Autodesk Inventor part; units mm, degrees
ref_plane "YZ Plane" through (0, 0, 0) normal (1, 0, 0) x (0, 1, 0)
ref_plane "XZ Plane" through (0, 0, 0) normal (0, 1, 0) x (-1, 0, 0)
ref_plane "XY Plane" through (0, 0, 0) normal (0, 0, 1) x (1, 0, 0)
sketch "Sketch1" plane through (0, 0, 0) normal (1, 0, 0) x (0, 1, 0)
  line L0 (0, 3.25) -> (10, 3.25)
  line L1 (10, 3.25) -> (10, -3.25)
  line L2 (10, -3.25) -> (0, -3.25)
  line L3 (0, -3.25) -> (0, 3.25)
  line L4 (10, 1.6898) -> (6.2365, 3.25)
  line L5 (10, -1.7859) -> (6.2365, -3.25)
  point P0 (0, 0)
  dimension "d0" = 10
  dimension "d1" = 6.5
  dimension "d2" = 3.25
  dimension "d3" = 0
extrude "Extrusion1" add sketch "Sketch1" along normal blind 3.9 and the other way blind 1.5 contours L0 L4 L1 L5 L2 L3
sketch "Sketch2" plane through (-1.5, 0, -3.25) normal (0, -1, 0) x (1, 0, 0)
  circle A0 centre (1.5, 3.25) radius 0.425
  line L0 (0, 0) -> (0, 6.5)
  dimension "d7" = 0.85
  dimension "d12" = 1.5
extrude "Extrusion2" add sketch "Sketch2" along normal blind 3.6
sketch "Sketch3" plane through (-1.5, 10, 1.6898) normal (0, 1, 0) x (1, 0, 0)
  circle A0 centre (1.5, 1.6898) radius 0.8517
extrude "Extrusion3" cut sketch "Sketch3" against normal blind 1
sketch "Sketch4" plane through (-1.5, 0, 3.25) normal (0, 0, 1) x (1, 0, 0)
  line L0 (0.648, 5.5866) -> (2.3749, 5.5866)
  line L1 (2.3749, 5.5866) -> (2.3749, 1.0456)
  line L2 (2.3749, 1.0456) -> (0.648, 1.0456)
  line L3 (0.648, 1.0456) -> (0.648, 5.5866)
  point P0 (1.5, 0)
extrude "Extrusion4" cut sketch "Sketch4" against normal blind 1
pattern_linear "Rectangular Pattern1" count 2 spacing 2.54 along (1, 0, 0) of "Extrusion4", "Extrusion3", "Extrusion2"
properties part number "Screw_Terminal_2Pos"
Verification items for the finished model (mm, model axes). A direction names the side the tool comes from. Coordinates: 2 decimals unless noted, no trailing zeros. Order: outer loops, then holes, each group sorted by start corner. A loop starts at its lowest first (then second) coordinate and runs counter-clockwise, first axis right, second up. Notation, with made-up numbers: (-3.5, -38.5) -> (33.5, -38.5) arc R22 ccw to (33.5, -22.5) -> close; hole circle Ø2 at (74, 46). An arc over 180 degrees is marked (long way). Use CSV: the item, a comma, the result in double quotes. Start each with the question number.
Q1. Section check C-C, the plane z = 2.75. Record the cut outline in (x, y).
Q2. Tool access check on faces 1 (the flat face through (2.5, -3.6, 0)), 2 (the flat face through (3.415, 3, 3)). Record the directions out of +Z, -Z, +X, -X, +Y, -Y that give a thin tool (end or side, any length) a straight path to the whole face; none if there is none.
Q3. Depth check by flat-ended pin: P1, Ø0.5, axis at x = 0.5, y = 2, coming from the +Z side; P2, Ø0.8, axis at x = 2.5, z = 2.5, coming from the +Y side; P3, Ø0.8, axis at x = 0, z = 2.5, coming from the -Y side. Enter the tip coordinate at first touch or a pass-through.
Q4. Draft check along Z on faces 3 (the cylindrical face through (2.115, -1.775, -0.019)), 4 (the cylindrical face through (-0.111, 9.507, -0.844)), 5 (the flat face through (3.9, 5, 0)). Enter one of: +Z half, -Z half, draft (parallel to the pull), parting line (faces both ways), or undercut.
Q5. Section check A-A, the plane y = -1.75. Record the cut outline in (x, z) (3 decimals).
Q6. Thickness scan on line 1 along X through (y, z) = (9.4, 0); line 2 along Y through (x, z) = (2.35, -0.5); line 3 along Z through (x, y) = (-0.5, 4.25). Record the ranges inside material, lowest first.
Q7. Section check D-D, the plane y = 8.25. Record the cut outline in (x, z).
Returned:
1,outline,"(-1.5, 0) -> (3.9, 0) -> (3.9, 7.44) -> (-1.5, 7.44) -> close; hole (-0.85, 1.05) -> (0.87, 1.05) -> (0.87, 5.59) -> (-0.85, 5.59) -> close; hole (1.69, 1.05) -> (3.41, 1.05) -> (3.41, 5.59) -> (1.69, 5.59) -> close"
2,face 1,"+Z, -Z, +X, -X, -Y"
2,face 2,"+Z"
3,P1,"stops at z = 2.25"
3,P2,"stops at y = 9.01"
3,P3,"stops at y = 0"
4,face 3,"parting line"
4,face 4,"undercut"
4,face 5,"draft"
5,outline,"circle Ø0.85 at (0, 0); circle Ø0.85 at (2.54, 0)"
6,line 1,"x = -1.5 to -0.85, 0.85 to 1.69, 3.39 to 3.9"
6,line 2,"y = 0 to 9"
6,line 3,"z = -3.25 to 2.25"
7,outline,"(-1.5, -2.47) -> (3.9, -2.47) -> (3.9, 2.42) -> (-1.5, 2.42) -> close"
